Read the model definition and answer for the solid it produces. Units are mm, in the model's axes. Give positions to 0.01 mm unless a question says otherwise; leave off trailing zeros. Order: outer loops, then holes, each group sorted by start corner. A loop starts at its lowest first (then second) coordinate and runs counter-clockwise, first axis right, second up. Notation, with made-up numbers: (73, 51.25) -> (111, 51.25) arc R12 ccw to (111, 70.25) -> close; hole circle Ø2 at (71, 4.25). An arc over 180 degrees is marked (long way). Answer as CSV lines item,"result". Start each with the question number.
1) Find section C-C (z = -13). Determine the outline of the cut face in (x, y), and give its area (3 significant figures).
2) Find section A-A (x = 0.5). Determine the outline of the cut face in (y, z).
3) Find section D-D (x = -6.25). Determine the outline of the cut face in (y, z).
4) Find section B-B (y = 1.85). Determine the outline of the cut face in (x, z), and give its area (3 significant figures).
5) Straight lines are drawn through the part: L1, parallel to Z at x = -0.5, y = 2.8; L2, parallel to Z at x = 1, y = 1.6; L3, parallel to X at y = 0.85, z = -12. For each, find the intervals that lie inside material, in ascending order. Write a range as from..to.
6) Flat-ended cylindrical pins translate along their axes: pin 1 Ø2.5 at (x, z) = (0, -8.27) entering from -Y; pin 2 Ø1 at (y, z) = (1.5, -35) entering from +X; pin 3 Ø0.9 at (y, z) = (1.5, -25.5) entering from -X; pin 4 Ø0.9 at (x, y) = (-7, 1.5) entering from +Z. Find the tip coordinate at first contact, or state that the pin passes through.
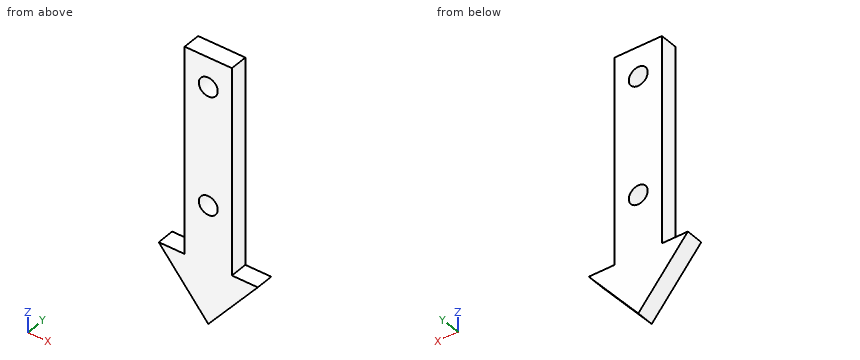
```python
from build123d import *

# Parameters (mm, degrees)
SKETCH1_R           = 1.6
BOSS_EXTRUDE1_DEPTH = 3


with BuildPart() as part:
    # Sketch1 → Boss-Extrude1 (new body)
    with BuildSketch(Plane(origin=(0, 0, 0), x_dir=(1, 0, 0), z_dir=(0, 1, 0))):
        Polygon((8.390996312, 38.269741393), (0, 48.269741393), (-8.390996312, 38.269741393), (-4, 38.269741393), (-4, 3.269741393), (4, 3.269741393), (4, 38.269741393), align=None)
        with Locations((0, 28.269741393)):
            Circle(SKETCH1_R, mode=Mode.SUBTRACT)
        with Locations((0, 8.269741393)):
            Circle(SKETCH1_R, mode=Mode.SUBTRACT)
    extrude(amount=BOSS_EXTRUDE1_DEPTH)


solid = part.part
```
Findings below:
1,outline,"(-4, 0) -> (4, 0) -> (4, 3) -> (-4, 3) -> close"
1,area,"24.0 mm²"
2,outline,"(0, -47.67) -> (3, -47.67) -> (3, -29.79) -> (0, -29.79) -> close; (0, -26.75) -> (3, -26.75) -> (3, -9.79) -> (0, -9.79) -> close; (0, -6.75) -> (3, -6.75) -> (3, -3.27) -> (0, -3.27) -> close"
3,outline,"(0, -40.82) -> (3, -40.82) -> (3, -38.27) -> (0, -38.27) -> close"
4,outline,"(-8.39, -38.27) -> (0, -48.27) -> (8.39, -38.27) -> (4, -38.27) -> (4, -3.27) -> (-4, -3.27) -> (-4, -38.27) -> close; hole circle Ø3.2 at (0, -28.27); hole circle Ø3.2 at (0, -8.27)"
4,area,"348 mm²"
5,L1,"-47.67..-29.79, -26.75..-9.79, -6.75..-3.27"
5,L2,"-47.08..-29.52, -27.02..-9.52, -7.02..-3.27"
5,L3,"-4..4"
6,pin 1,"through"
6,pin 2,"x = 4"
6,pin 3,"x = -4"
6,pin 4,"z = -38.27"
